Input: part model. Units: mm. Frame: model coordinates. A direction names the side the tool comes from. Coordinates: 2 decimals unless noted, no trailing zeros. Loops run counter-clockwise (first coordinate to the right, second up) from the corner with the lowest first, then second, coordinate; pieces in that order, holes last.
(1) Mould query, pull axis X, two halves, no side actions, for faces 1 (the face through (0, 12.9, -16)), 2 (the face through (10, 4, -23)), 3 (the face through (210, 4, -30)), 4 (the face through (10, 4, 22)). Classes: released by +X, released by -X, zero draft, split by the parting line, or undercut.
(2) Contact query for flat-ended pins moving along their axis: P1, Ø6.5, axis at x = -1, z = -15, coming from the +Y side; P2, Ø4, axis at x = 189, y = 4, coming from the +Z side; P3, Ø5, axis at y = 11, z = 9, coming from the -X side; P4, Ø4.5, axis at x = 60, z = 9, coming from the +Y side. Output: stop coordinate, or through.
(3) Line query: L1, parallel to Z at x = 60, y = 6.5 (3 decimals); L2, parallel to Y at x = 237, z = -42; L3, parallel to Y at x = 89, z = 7. Output: solid intervals per line, ascending.
(4) Section A-A, the plane y = 10.75. Return loops of the section in (x, z) (3 decimals).
(5) Section D-D, the plane x = 50. Return loops of the section in (y, z), then the cut area to 3 significant figures.
(6) Section B-B, the plane x = 0. Return loops of the section in (y, z).
(7) Section C-C, the plane z = 4. Return loops of the section in (x, y), then the cut area to 3 significant figures.
(8) Set-up query: faces 5 (the face through (-0.63, 10.42, -18.33)), 6 (the face through (0, 4, -30)), 7 (the face through (161, 8, -1)), 8 (the face through (20, 11, 0)). Return all of +Z, -Z, +X, -X, +Y, -Y with unobstructed straight access to the full face (end or side cutting, diameter ignored); none if empty.
Autodesk Inventor part; units mm, degrees
ref_plane "YZ Plane" through (0, 0, 0) normal (1, 0, 0) x (0, 1, 0)
ref_plane "XZ Plane" through (0, 0, 0) normal (0, 1, 0) x (-1, 0, 0)
ref_plane "XY Plane" through (0, 0, 0) normal (0, 0, 1) x (1, 0, 0)
sketch "Sketch1" plane through (0, 0, 0) normal (0, 1, 0) x (-1, 0, 0)
  line L0 (10, 30) -> (10, -30)
  line L1 (10, -30) -> (-10, -30)
  line L2 (-10, -30) -> (-10, -15)
  line L3 (-10, -15) -> (-230, -15)
  line L4 (-230, -15) -> (-230, 15)
  line L5 (-230, 15) -> (-10, 15)
  line L6 (-10, 15) -> (-10, 30)
  line L7 (-10, 30) -> (10, 30)
  line L8 (58, 0) -> (-278, 0) construction
  point P0 (0, 0)
  dimension "d0" = 60
  dimension "d2" = 10
  dimension "d3" = 10
  dimension "d4" = 30
  dimension "d5" = 220
extrude "Extrusion1" add sketch "Sketch1" along normal blind 8
sketch "Sketch2" plane through (0, 8, 0) normal (0, 1, 0) x (1, 0, 0)
  circle A0 centre (0, -15.5) radius 2.9
  circle A1 centre (0, 15.5) radius 2.9
  line L0 (0, 42) -> (0, -42) construction
  line L1 (-58, 0) -> (278, 0) construction
  point P0 (0, 0)
  dimension "d8" = 5.8
  dimension "d9" = 31
extrude "Extrusion2" add sketch "Sketch2" along normal blind 4.9
sketch "Sketch3" plane through (0, 8, 0) normal (0, 1, 0) x (1, 0, 0)
  line L0 (230, 15) -> (10, 15) construction
  line L1 (10, -15) -> (230, -15) construction
  line L2 (20, 15) -> (70, 15)
  line L3 (70, 15) -> (70, -15)
  line L4 (70, -15) -> (20, -15)
  line L5 (20, -15) -> (20, 15)
  point P0 (0, 0)
  dimension "d12" = 10
  dimension "d13" = 50
extrude "Extrusion3" add sketch "Sketch3" along normal blind 5.1
sketch "Sketch4" plane through (0, 13.1, 0) normal (0, 1, 0) x (1, 0, 0)
  circle A0 centre (35, 9) radius 1.475
  circle A1 centre (60, 9) radius 1.475
  circle A2 centre (35, -9) radius 1.475
  circle A3 centre (60, -9) radius 1.475
  line L0 (-58, 0) -> (278, 0) construction
  line L1 (35, 9) -> (35, -9) construction
  line L2 (60, 9) -> (60, -9) construction
  line L3 (20, 15) -> (20, -15) construction
  point P0 (0, 0)
  dimension "d16" = 2.95
  dimension "d17" = 18
  dimension "d18" = 25
  dimension "d19" = 15
extrude "Extrusion4" cut sketch "Sketch4" against normal up to surface (13.1 mm away)
sketch "Sketch7" plane through (230, 0, -15) normal (0, 0, -1) x (-1, 0, 0)
  line L0 (0, 0) -> (0, 8)
  line L1 (0, 8) -> (160, 8)
  line L2 (0, 0) -> (220, 0)
  line L3 (20, 0) -> (20, 8)
  point P0 (230, 0)
  dimension "d37" = 20
extrude "Extrusion7" add sketch "Sketch7" along normal blind 29.5
sketch "Sketch8" plane through (230, 0, 15) normal (1, 0, 0) x (0, 0, -1)
  line L0 (0, 0) -> (0, 8)
  line L1 (59.5, 8) -> (59.5, 0)
  line L2 (0, 0) -> (59.5, 0)
  line L3 (0, 8) -> (59.5, 8)
  line L4 (4, 8) -> (4, 0)
  line L5 (55.5, 8) -> (55.5, 0)
  point P0 (15, 0)
  dimension "d40" = 4
  dimension "d41" = 4
extrude "Extrusion8" add sketch "Sketch8" along normal blind 26 contours L0 L3 L4 L2 | L5 L3 L1 L2
sketch "Sketch9" plane through (10, 0, 15) normal (0, 0, 1) x (1, 0, 0)
  line L0 (246, 8) -> (246, 0) construction
  line L1 (246, 4) -> (227, 4) construction
  circle A0 centre (227, 4) radius 2
  circle A1 centre (235, 4) radius 2
  circle A2 centre (243, 4) radius 2
  point P0 (-10, 0)
  dimension "d44" = 4
  dimension "d45" = 8
  dimension "d46" = 8
  dimension "d47" = 3
extrude "Extrusion9" cut sketch "Sketch9" against normal up to surface (59.5 mm away)
fillet "Fillet4" radius 3 2 edges at (210, 4, -15) (210, 4, -44.5)
fillet "Fillet5" radius 3 6 edges at (230, 0, -14.75) (230, 8, -14.75) (256, 0, 13) (256, 8, 13) (256, 0, -42.5) (256, 8, -42.5)
fillet "Fillet2" radius 3 4 edges at (20, 10.55, 15) (20, 10.55, -15) (70, 10.55, 15) (70, 10.55, -15)
fillet "Fillet3" radius 3 6 edges at (10, 4, 15) (10, 4, 30) (-10, 4, 30) (-10, 4, -30) (10, 4, -30) (10, 4, -15)
properties part number "Arm"
Report:
1. face 1: zero draft
1. face 2: undercut
1. face 3: undercut
1. face 4: released by +X
2. P1: stops at y = 12.9
2. P2: stops at z = 15
2. P3: stops at x = 20
2. P4: stops at y = 13.1
3. L1: z = -15 to -10.475, -7.525 to 7.525, 10.475 to 15
3. L2: y = 0 to 2, 6 to 8
3. L3: y = 0 to 8
4. outline: circle Ø5.8 at (0, -15.5); circle Ø5.8 at (0, 15.5); (20, -12) arc R3 ccw to (23, -15) - (67, -15) arc R3 ccw to (70, -12) - (70, 12) arc R3 ccw to (67, 15) - (23, 15) arc R3 ccw to (20, 12) - close; hole circle Ø2.95 at (35, -9); hole circle Ø2.95 at (35, 9); hole circle Ø2.95 at (60, -9); hole circle Ø2.95 at (60, 9)
5. outline: (0, -15) - (13.1, -15) - (13.1, 15) - (0, 15) - close
5. area: 393 mm2
6. outline: (0, -30) - (8, -30) - (8, -18.4) - (12.9, -18.4) - (12.9, -12.6) - (8, -12.6) - (8, 12.6) - (12.9, 12.6) - (12.9, 18.4) - (8, 18.4) - (8, 30) - (0, 30) - close
7. outline: (-10, 0) - (227, 0) arc R3 ccw to (230, 3) - (230, 5) arc R3 ccw to (227, 8) - (70, 8) - (70, 13.1) - (20, 13.1) - (20, 8) - (-10, 8) - close
7. area: 2,170 mm2
8. face 5: +Y
8. face 6: -Z, -X, +Y, -Y
8. face 7: +Z, -Z, +X, +Y
8. face 8: +Z, -Z, -X, +Y
